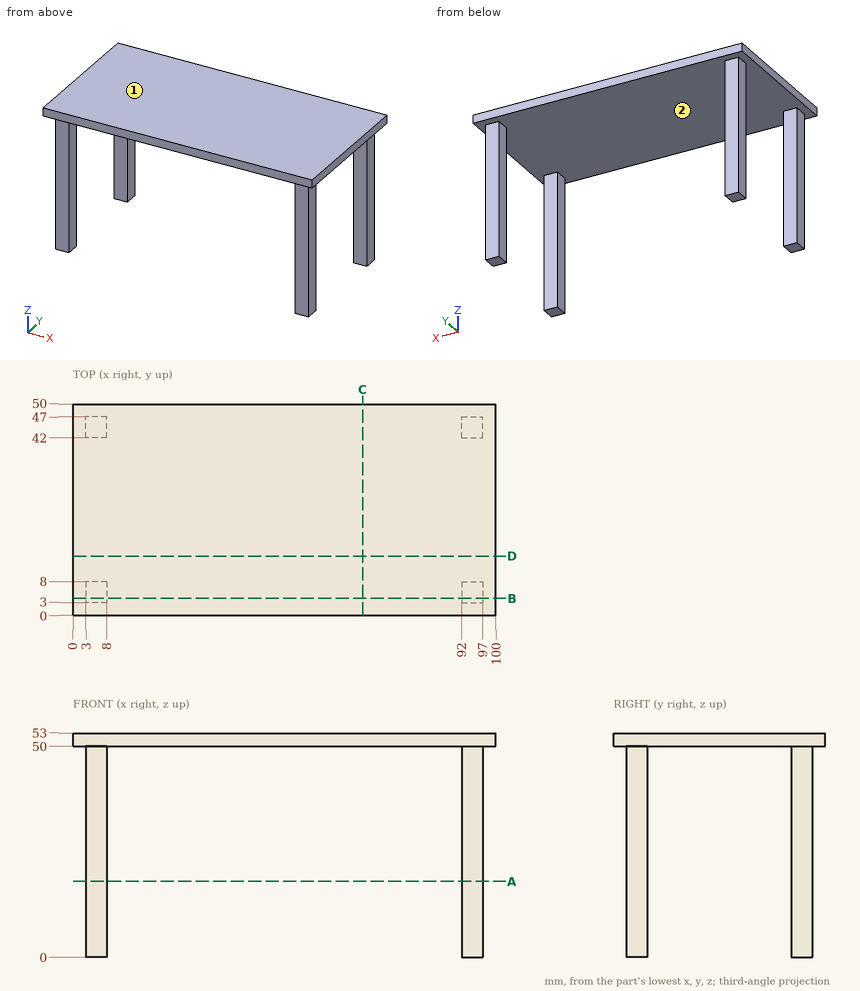
Verification items for this drawing (mm, ordinates from the low corner). Round coordinates to 2 decimals unless told otherwise and drop trailing zeros. Loops run counter-clockwise (first coordinate to the right, second up) from the corner with the lowest first, then second, coordinate; pieces in that order, holes last. Notation, with made-up numbers: M 83.25,80 L 108.25,80 A35 ccw 108.25,119 Z; hole C -21,37.5 d11. An arc over 180 degrees is marked long. Answer as a JSON object with one key per item and string values.
1. Section check B-B (y = 4). Record the boundary of the cut face in (x, z).
Reply:
{"outline": "M 0,50 L 3,50 L 3,0 L 8,0 L 8,50 L 92,50 L 92,0 L 97,0 L 97,50 L 100,50 L 100,53 L 0,53 Z"}
2. Gauge pin test, flat ends, axial feed: P1, Ø8, axis at y = 44, z = 17, coming from the +X side; P2, Ø6, axis at x = 41, y = 9, coming from the -Z side; P3, Ø5.5, axis at x = 5.5, z = 33, coming from the -Y side. Record the tip position at first contact, or that the pin passes through.
Reply:
{"P1": "stops at x = 97", "P2": "stops at z = 50", "P3": "stops at y = 3"}
3. Scan lines: line 1 (X direction, y = 45.5, z = 9); line 2 (Z direction, x = 93.5, y = 31.5). Record each from-to range of solid material in increasing order.
Reply:
{"line 1": "x = 3 to 8, 92 to 97", "line 2": "z = 50 to 53"}
4. Section check C-C (x = 68.5). Record the boundary of the cut face in (y, z), plus the area to 3 significant figures.
Reply:
{"outline": "M 0,50 L 50,50 L 50,53 L 0,53 Z", "area": "150 mm²"}
5. Section check A-A (z = 18). Record the boundary of the cut face in (x, y).
Reply:
{"outline": "M 3,3 L 8,3 L 8,8 L 3,8 Z; M 3,42 L 8,42 L 8,47 L 3,47 Z; M 92,3 L 97,3 L 97,8 L 92,8 Z; M 92,42 L 97,42 L 97,47 L 92,47 Z"}
6. Mould release check, pull along X, two halves, no side actions. Record for the marked faces 1 and 2: pulls with the +X half, pulls with the -X half, needs draft (parallel to the pull), parting line crosses it, or undercut.
Reply:
{"face 1": "needs draft", "face 2": "undercut"}
7. Section check D-D (y = 14). Record the boundary of the cut face in (x, z), plus the area to 3 significant figures.
Reply:
{"outline": "M 0,50 L 100,50 L 100,53 L 0,53 Z", "area": "300 mm²"}
